```python
from build123d import *

# Parameters (mm, degrees)
PAD_DEPTH          = 9
SKETCH001_W        = 26.1
SKETCH001_H        = 34.4
POCKET_DEPTH       = 3
SKETCH002_R        = 22.22
PAD001_DEPTH       = 3
SKETCH003_R        = 24.44
PAD002_DEPTH       = 3
SKETCH004_R        = 26.6
PAD003_DEPTH       = 3
SKETCH005_R        = 28
PAD004_DEPTH       = 3
SKETCH006_R        = 29
PAD005_DEPTH       = 3
SKETCH007_R        = 29
PAD006_DEPTH       = 3
SKETCH008_R        = 29
PAD007_DEPTH       = 3
SKETCH009_W        = 17
SKETCH009_H        = 24
POCKET001_DEPTH    = 3
SKETCH010_W        = 16
SKETCH010_H        = 9
POCKET002_DEPTH    = 7
SKETCH011_W        = 20
SKETCH011_H        = 9
POCKET003_DEPTH    = 3
SKETCH012_R        = 1.25
POCKET004_DEPTH    = 270.433943
POLARPATTERN_COUNT = 6
SKETCH013_W        = 3
SKETCH013_H        = 38
POCKET005_DEPTH    = 3
SKETCH014_W        = 3
SKETCH014_H        = 6
POCKET006_DEPTH    = 6
SKETCH015_W        = 10.05
SKETCH015_H        = 6
POCKET007_DEPTH    = 3
FILLET_R           = 4
FILLET001_R        = 3
FILLET002_R        = 3
FILLET003_R        = 3
FILLET004_R        = 3


with BuildPart() as part:
    # Sketch → Pad (new body)
    with BuildSketch(Plane.XY):
        Polygon((44, 0), (22, 38.105118), (-22, 38.105118), (-44, 0), (-22, -38.105118), (22, -38.105118), align=None)
    extrude(amount=PAD_DEPTH)

    # Sketch001 (on Face8 of Pad) → Pocket (cut)
    with BuildSketch(Plane.XY.offset(9)):
        with Locations((0, -13.905118)):
            Rectangle(SKETCH001_W, SKETCH001_H)
    extrude(amount=-POCKET_DEPTH, mode=Mode.SUBTRACT)

    # Sketch002 (on Face5 of Pocket) → Pad001 (join)
    with BuildSketch(Plane.XY.offset(9)):
        Polygon((22, 38.105118), (-22, 38.105118), (-44, 0), (-22, -38.105118), (22, -38.105118), (44, 0), align=None)
        Circle(SKETCH002_R, mode=Mode.SUBTRACT)
    extrude(amount=PAD001_DEPTH)

    # Sketch003 (on Face14 of Pad001) → Pad002 (join)
    with BuildSketch(Plane.XY.offset(12)):
        Polygon((40, 0), (20, 34.641016), (-20, 34.641016), (-40, 0), (-20, -34.641016), (20, -34.641016), align=None)
        Circle(SKETCH003_R, mode=Mode.SUBTRACT)
    extrude(amount=PAD002_DEPTH)

    # Sketch004 (on Face21 of Pad002) → Pad003 (join)
    with BuildSketch(Plane.XY.offset(15)):
        Polygon((41, 0), (20.5, 35.507042), (-20.5, 35.507042), (-41, 0), (-20.5, -35.507042), (20.5, -35.507042), align=None)
        Circle(SKETCH004_R, mode=Mode.SUBTRACT)
    extrude(amount=PAD003_DEPTH)

    # Sketch005 (on Face28 of Pad003) → Pad004 (join)
    with BuildSketch(Plane.XY.offset(18)):
        Polygon((19, 32.908965), (-19, 32.908965), (-38, 0), (-19, -32.908965), (19, -32.908965), (38, 0), align=None)
        Circle(SKETCH005_R, mode=Mode.SUBTRACT)
    extrude(amount=PAD004_DEPTH)

    # Sketch006 (on Face35 of Pad004) → Pad005 (join)
    with BuildSketch(Plane.XY.offset(21)):
        Polygon((39, 0), (19.5, 33.774991), (-19.5, 33.774991), (-39, 0), (-19.5, -33.774991), (19.5, -33.774991), align=None)
        Circle(SKETCH006_R, mode=Mode.SUBTRACT)
    extrude(amount=PAD005_DEPTH)

    # Sketch007 (on Face42 of Pad005) → Pad006 (join)
    with BuildSketch(Plane.XY.offset(24)):
        Polygon((36, 0), (18, 31.176915), (-18, 31.176915), (-36, 0), (-18, -31.176915), (18, -31.176915), align=None)
        Circle(SKETCH007_R, mode=Mode.SUBTRACT)
    extrude(amount=PAD006_DEPTH)

    # Sketch008 (on Face49 of Pad006) → Pad007 (join)
    with BuildSketch(Plane.XY.offset(27)):
        Polygon((37, 0), (18.5, 32.04294), (-18.5, 32.04294), (-37, 0), (-18.5, -32.04294), (18.5, -32.04294), align=None)
        Circle(SKETCH008_R, mode=Mode.SUBTRACT)
    extrude(amount=PAD007_DEPTH)

    # Sketch009 (on Face74 of Pad007) → Pocket001 (cut)
    with BuildSketch(Plane.XY.offset(6)):
        with Locations((0, -8.705118)):
            Rectangle(SKETCH009_W, SKETCH009_H)
    extrude(amount=-POCKET001_DEPTH, mode=Mode.SUBTRACT)

    # Sketch010 (on Face12 of Pocket001) → Pocket002 (cut)
    with BuildSketch(Plane.XZ.offset(38.105118)):
        with Locations((0, 7.5)):
            Rectangle(SKETCH010_W, SKETCH010_H)
    extrude(amount=-POCKET002_DEPTH, mode=Mode.SUBTRACT)

    # Sketch011 (on Face40 of Pocket002) → Pocket003 (cut)
    with BuildSketch(Plane.XY.offset(9)):
        with Locations((0, 17.72)):
            Rectangle(SKETCH011_W, SKETCH011_H)
    extrude(amount=-POCKET003_DEPTH, mode=Mode.SUBTRACT)

    # Sketch012 (on Face93 of Pocket003) → Pocket004 (cut, through all)
    with BuildSketch(Plane.XY.offset(30)):
        with Locations((-32.33, 0)):
            Circle(SKETCH012_R)
    pocket004 = extrude(amount=-POCKET004_DEPTH, mode=Mode.SUBTRACT)

    # PolarPattern: Pocket004 ×6 about axis
    polarpattern_axis = Axis((0, 0, 30), (0, 0, 1))
    for i in range(1, POLARPATTERN_COUNT):
        add(pocket004.rotate(polarpattern_axis, i * 360 / POLARPATTERN_COUNT), mode=Mode.SUBTRACT)

    # Sketch013 (on Face45 of PolarPattern) → Pocket005 (cut)
    with BuildSketch(Plane.XY.offset(6)):
        with Locations((-11.55, -12.105118)):
            Rectangle(SKETCH013_W, SKETCH013_H)
    extrude(amount=-POCKET005_DEPTH, mode=Mode.SUBTRACT)

    # Sketch014 (on Face58 of Pocket005) → Pocket006 (cut)
    with BuildSketch(Plane.XY.offset(9)):
        with Locations((-11.55, 6.294882)):
            Rectangle(SKETCH014_W, SKETCH014_H)
    extrude(amount=-POCKET006_DEPTH, mode=Mode.SUBTRACT)

    # Sketch015 (on Face58 of Pocket006) → Pocket007 (cut)
    with BuildSketch(Plane.XY.offset(9)):
        with Locations((-5.025, 6.294882)):
            Rectangle(SKETCH015_W, SKETCH015_H)
    extrude(amount=-POCKET007_DEPTH, mode=Mode.SUBTRACT)

    # Fillet
    fillet_edges = [part.edges().sort_by_distance(p)[0] for p in [
        (22, -38.105118, 4.5),
        (44, 0, 4.5),
        (22, 38.105118, 4.5),
        (-22, 38.105118, 4.5),
        (-44, 0, 4.5),
        (-22, -38.105118, 4.5),
    ]]
    fillet(fillet_edges, radius=FILLET_R)

    # Fillet001
    fillet001_edges = [part.edges().sort_by_distance(p)[0] for p in [
        (20.5, -35.507042, 16.5),
        (41, 0, 16.5),
        (20.5, 35.507042, 16.5),
        (-20.5, 35.507042, 16.5),
        (-41, 0, 16.5),
        (-20.5, -35.507042, 16.5),
    ]]
    fillet(fillet001_edges, radius=FILLET001_R)

    # Fillet002
    fillet002_edges = [part.edges().sort_by_distance(p)[0] for p in [
        (19.5, -33.774991, 22.5),
        (-19.5, -33.774991, 22.5),
        (-39, 0, 22.5),
        (-19.5, 33.774991, 22.5),
        (19.5, 33.774991, 22.5),
        (39, 0, 22.5),
    ]]
    fillet(fillet002_edges, radius=FILLET002_R)

    # Fillet003
    fillet003_edges = [part.edges().sort_by_distance(p)[0] for p in [
        (-18.5, -32.04294, 28.5),
        (18.5, -32.04294, 28.5),
        (37, 0, 28.5),
        (-37, 0, 28.5),
        (18.5, 32.04294, 28.5),
        (-18.5, 32.04294, 28.5),
    ]]
    fillet(fillet003_edges, radius=FILLET003_R)

    # Fillet004
    fillet004_edges = [part.edges().sort_by_distance(p)[0] for p in [
        (-20, -34.641016, 13.5),
        (20, -34.641016, 13.5),
        (40, 0, 13.5),
        (-40, 0, 13.5),
        (-38, 0, 19.5),
        (-19, -32.908965, 19.5),
        (19, -32.908965, 19.5),
        (38, 0, 19.5),
        (36, 0, 25.5),
        (18, -31.176915, 25.5),
        (-18, -31.176915, 25.5),
        (-36, 0, 25.5),
        (18, 31.176915, 25.5),
        (-18, 31.176915, 25.5),
        (-19, 32.908965, 19.5),
        (-20, 34.641016, 13.5),
        (20, 34.641016, 13.5),
        (19, 32.908965, 19.5),
    ]]
    fillet(fillet004_edges, radius=FILLET004_R)


solid = part.part
```
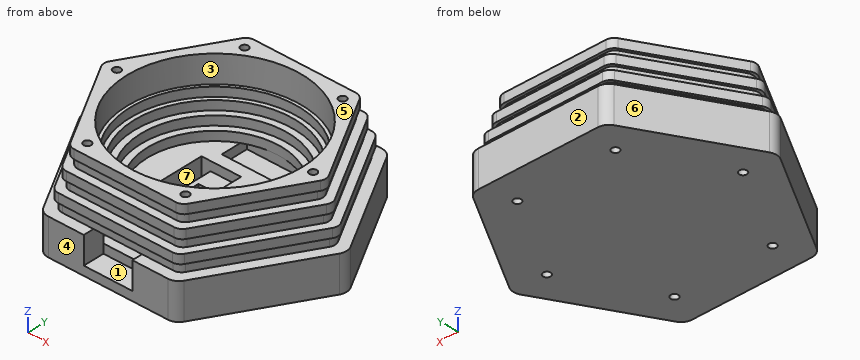
Work out the finished part from the listing and answer in its coordinate system (mm). Face numbers are marked on the shaded views. A direction names the side the tool comes from. Round coordinates to 2 decimals unless told otherwise and drop trailing zeros. Loops run counter-clockwise (first coordinate to the right, second up) from the corner with the lowest first, then second, coordinate; pieces in that order, holes last.
(1) The mould has two halves that part along Y. Classify the marked faces 4, 5, 6 and 7: pulls with the +Y half, pulls with the -Y half, needs draft (parallel to the pull), parting line crosses it, or undercut.
Computed values:
face 4: pulls with the -Y half
face 5: needs draft
face 6: pulls with the +Y half
face 7: undercut
(2) The part is cut by section D-D, the plane z = 19.25. Give the vertices of the cut face in (x, y) (3 decimals), and give its area (3 significant figures).
Computed values:
outline: (-37.134, -1.5) - (-19.866, -31.409) arc R3 ccw to (-17.268, -32.909) - (17.268, -32.909) arc R3 ccw to (19.866, -31.409) - (37.134, -1.5) arc R3 ccw to (37.134, 1.5) - (19.866, 31.409) arc R3 ccw to (17.268, 32.909) - (-17.268, 32.909) arc R3 ccw to (-19.866, 31.409) - (-37.134, 1.5) arc R3 ccw to start; hole circle Ø2.5 at (-32.33, 0); hole circle Ø56 at (0, 0); hole circle Ø2.5 at (-16.165, -27.999); hole circle Ø2.5 at (-16.165, 27.999); hole circle Ø2.5 at (16.165, -27.999); hole circle Ø2.5 at (16.165, 27.999); hole circle Ø2.5 at (32.33, 0)
area: 1,260 mm2
(3) The part is cut by section B-B, the plane y = 0. Give the number of separate pieces and of enclosed holes in the cut face, and give its area (3 significant figures).
Computed values:
separate pieces: 3
enclosed holes: 0
area: 993 mm2
(4) Find the intervals of material crossed by L1, parallel to Y at x = -16, z = 8; L2, parallel to Z at x = -9, y = -22.5; L3, parallel to Z at x = 1, y = -32.5, in increasing order.
Computed values:
L1: y = -38.11 to -29.24, -26.76 to 26.76, 29.24 to 38.11
L2: z = 0 to 6, 9 to 12
L3: z = 0 to 3, 12 to 24
(5) The part is cut by section A-A, the plane z = 25.5. Give the vertices of the cut face in (x, y) (3 decimals), and give its area (3 significant figures).
Computed values:
outline: (-35.134, -1.5) - (-18.866, -29.677) arc R3 ccw to (-16.268, -31.177) - (16.268, -31.177) arc R3 ccw to (18.866, -29.677) - (35.134, -1.5) arc R3 ccw to (35.134, 1.5) - (18.866, 29.677) arc R3 ccw to (16.268, 31.177) - (-16.268, 31.177) arc R3 ccw to (-18.866, 29.677) - (-35.134, 1.5) arc R3 ccw to start; hole circle Ø2.5 at (-32.33, 0); hole circle Ø58 at (0, 0); hole circle Ø2.5 at (-16.165, -27.999); hole circle Ø2.5 at (-16.165, 27.999); hole circle Ø2.5 at (16.165, -27.999); hole circle Ø2.5 at (16.165, 27.999); hole circle Ø2.5 at (32.33, 0)
area: 693 mm2
(6) For the marked faces 1, 2 and 3, determine the directions among +Z, -Z, +X, -X, +Y, -Y from which every point of the face is accessible in a straight line to the end or side of a thin tool.
Computed values:
face 1: -Y
face 2: +Z, -Z, +X, -X, +Y
face 3: +Z
(7) Each of these flat-tipped pins is pushed along its axis until it touches: P1, Ø3, axis at x = -24.5, z = 4.5, coming from the +Y side; P2, Ø0.9, axis at x = 3, z = 25, coming from the +Y side; P3, Ø5.5, axis at y = -33.5, z = 7, coming from the -X side. Where does it stop, or does it pass through?
Computed values:
P1: stops at y = 36.35
P2: stops at y = 31.18
P3: stops at x = -26.25
